Verification items for this drawing (mm, ordinates from the low corner). Give positions to 0.01 mm unless a question says otherwise; leave off trailing zeros. Write each loop counter-clockwise with the first axis right and the second up, starting at its lowest first coordinate (ties: lowest second). Pieces come first, ordered by that corner, then holes. Notation, with made-up numbers: (-7.5, 55) -> (32.5, 55) arc R17 ccw to (32.5, 83) -> close; hole circle Ø5 at (75.5, -9.5). An arc over 180 degrees is marked (long way). Answer as a JSON object with one key per item and string values.
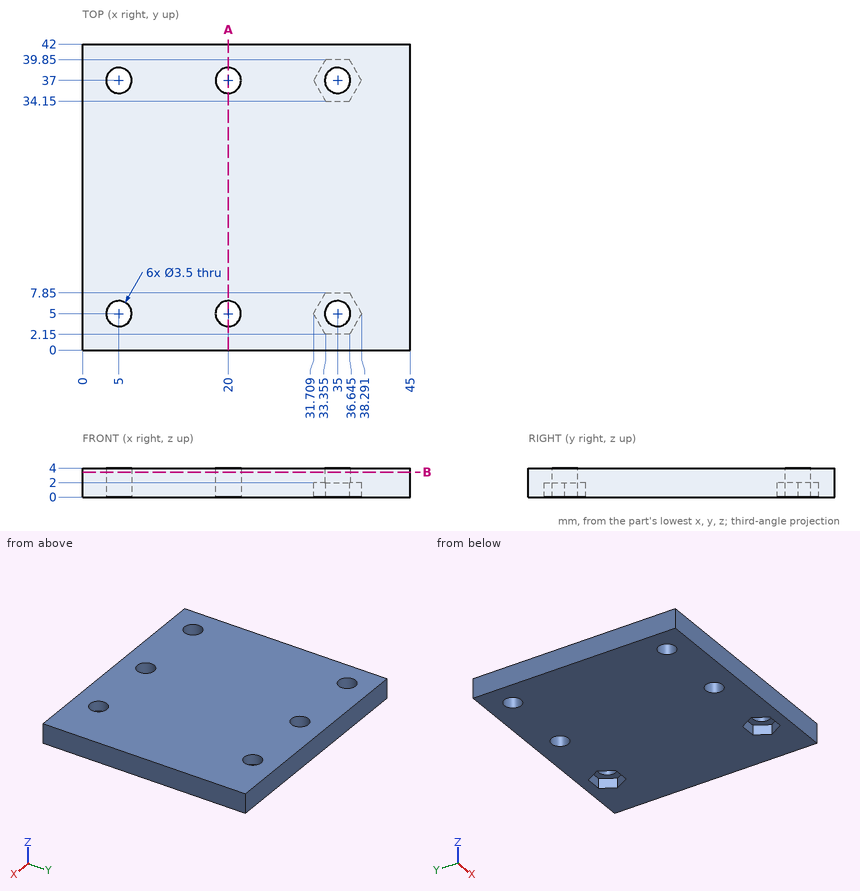
1. Sectioned sample at A-A, the plane x = 20. Enter the section's corners in (y, z).
Determined:
{"outline": "(0, 0) -> (3.25, 0) -> (3.25, 4) -> (0, 4) -> close; (6.75, 0) -> (35.25, 0) -> (35.25, 4) -> (6.75, 4) -> close; (38.75, 0) -> (42, 0) -> (42, 4) -> (38.75, 4) -> close"}
2. Sectioned sample at B-B, the plane z = 3.45. Enter the section's corners in (x, y).
Determined:
{"outline": "(0, 0) -> (45, 0) -> (45, 42) -> (0, 42) -> close; hole circle Ø3.5 at (5, 5); hole circle Ø3.5 at (5, 37); hole circle Ø3.5 at (20, 5); hole circle Ø3.5 at (20, 37); hole circle Ø3.5 at (35, 5); hole circle Ø3.5 at (35, 37)"}
3. Go/stop test with flat-tipped pins: P1, Ø0.6, axis at x = 35, z = 1, coming from the -Y side; P2, Ø5.5, axis at x = 35, y = 5, coming from the -Z side. Record where each tip stops, or that it passes through.
Determined:
{"P1": "y = 0", "P2": "z = 2"}
4. Scan lines: L1, parallel to Y at x = 5, z = 2; L2, parallel to X at y = 5, z = 1.6; L3, parallel to X at y = 5, z = 3.2. Record each from-to range of solid material in increasing order. Write a range as [from, to].
Determined:
{"L1": "[0, 3.25], [6.75, 35.25], [38.75, 42]", "L2": "[0, 3.25], [6.75, 18.25], [21.75, 31.71], [38.29, 45]", "L3": "[0, 3.25], [6.75, 18.25], [21.75, 33.25], [36.75, 45]"}
